from build123d import *

# Parameters (mm, degrees)
BOSS_EXTRUDE1_DEPTH = 15
HOLE1_D             = 51
HOLE2_D             = 14
HOLE2_DEPTH         = 15
HOLE3_D             = 20
HOLE3_DEPTH         = 15
FILLET1_R           = 2
CHAMFER1_SIZE       = 0.81
CHAMFER2_SIZE       = 2


with BuildPart() as part:
    # Sketch1 → Boss-Extrude1 (new body)
    with BuildSketch(Plane(origin=(0, 0, 0), x_dir=(0, 0, -1), z_dir=(1, 0, 0))):
        with BuildLine():
            Line((-62.994461331, 43.470654948), (-63.982276259, 1.506095834))
            ThreePointArc((-63.982276259, 1.506095834), (-64, 0), (-63.982276259, -1.506095834))
            Line((-63.982276259, -1.506095834), (-62.994461331, -43.470654948))
            ThreePointArc((-62.994461331, -43.470654948), (-57.142135624, -57.142135624), (-43.470654948, -62.994461331))
            Line((-43.470654948, -62.994461331), (-1.506095834, -63.982276259))
            ThreePointArc((-1.506095834, -63.982276259), (0, -64), (1.506095834, -63.982276259))
            Line((1.506095834, -63.982276259), (43.470654948, -62.994461331))
            ThreePointArc((43.470654948, -62.994461331), (57.142135624, -57.142135624), (62.994461331, -43.470654948))
            Line((62.994461331, -43.470654948), (63.982276259, -1.506095834))
            ThreePointArc((63.982276259, -1.506095834), (64, 0), (63.982276259, 1.506095834))
            Line((63.982276259, 1.506095834), (62.994461331, 43.470654948))
            ThreePointArc((62.994461331, 43.470654948), (57.142135624, 57.142135624), (43.470654948, 62.994461331))
            Line((43.470654948, 62.994461331), (1.506095834, 63.982276259))
            ThreePointArc((1.506095834, 63.982276259), (0, 64), (-1.506095834, 63.982276259))
            Line((-1.506095834, 63.982276259), (-43.470654948, 62.994461331))
            ThreePointArc((-43.470654948, 62.994461331), (-57.142135624, 57.142135624), (-62.994461331, 43.470654948))
        make_face()
    extrude(amount=-BOSS_EXTRUDE1_DEPTH)

    # Sketch2 → Revolve1 (revolve)
    with BuildSketch(Plane.XY, mode=Mode.PRIVATE) as revolve1_sk:
        Polygon((-15, 47.5), (-17, 45.5), (-17, 34.5), (-34, 34.5), (-50, 38.787187079), (-50, 76), (-65, 76), (-65, 48), (-67, 46), (-67, 0), (-15, 0), align=None)
    revolve(revolve1_sk.sketch.rotate(Axis((-67, 0, 0), (1, 0, 0)), 180), axis=Axis((-67, 0, 0), (1, 0, 0)))

    # Hole1 (through all)
    with Locations(Plane.ZY.offset(67)):
        with Locations((0, 0)):
            Hole(HOLE1_D / 2)

    # Hole2
    with Locations(Plane(origin=(0, 0, 0), x_dir=(0, 0, -1), z_dir=(1, 0, 0))):
        with Locations((43, 43), (43, -43), (-43, -43), (-43, 43)):
            Hole(HOLE2_D / 2, depth=HOLE2_DEPTH)

    # Hole3
    with Locations(Plane.ZY.offset(65)):
        with Locations((43, 43), (-43, 43), (-43, -43), (43, -43)):
            Hole(HOLE3_D / 2, depth=HOLE3_DEPTH)

    # Fillet1
    fillet1_edges = [part.edges().sort_by_distance(p)[0] for p in [
        (-17, 34.5, 0),
        (-50, 38.787187079, 0),
    ]]
    fillet(fillet1_edges, radius=FILLET1_R)

    # Chamfer1
    chamfer1_edges = [part.edges().sort_by_distance(p)[0] for p in [
        (-15, 0, -64),
        (0, -63.488368795, -22.488375391),
        (0, -64, 0),
        (0, -63.488368795, 22.488375391),
        (-15, 22.488375391, -63.488368795),
        (0, -57.142135624, 57.142135624),
        (0, -22.488375391, 63.488368795),
        (0, 0, 64),
        (0, 22.488375391, 63.488368795),
        (0, 57.142135624, 57.142135624),
        (0, 63.488368795, 22.488375391),
        (0, 64, 0),
        (0, 63.488368795, -22.488375391),
        (0, 57.142135624, -57.142135624),
        (0, 22.488375391, -63.488368795),
        (-15, 57.142135624, -57.142135624),
        (0, 0, -64),
        (0, -22.488375391, -63.488368795),
        (0, -57.142135624, -57.142135624),
        (-15, 63.488368795, -22.488375391),
        (-15, 64, 0),
        (-15, 63.488368795, 22.488375391),
        (-15, 57.142135624, 57.142135624),
        (-15, 22.488375391, 63.488368795),
        (-15, 0, 64),
        (-50, 76, 0),
        (-65, 76, 0),
        (-15, -22.488375391, 63.488368795),
        (-15, -57.142135624, -57.142135624),
        (-15, -57.142135624, 57.142135624),
        (-15, -63.488368795, 22.488375391),
        (-15, -64, 0),
        (-15, -63.488368795, -22.488375391),
        (-15, -22.488375391, -63.488368795),
    ]]
    chamfer(chamfer1_edges, length=CHAMFER1_SIZE)

    # Chamfer2
    chamfer2_edges = [part.edges().sort_by_distance(p)[0] for p in [
        (-67, 0, 25.5),
        (0, 0, 25.5),
    ]]
    chamfer(chamfer2_edges, length=CHAMFER2_SIZE)


solid = part.part
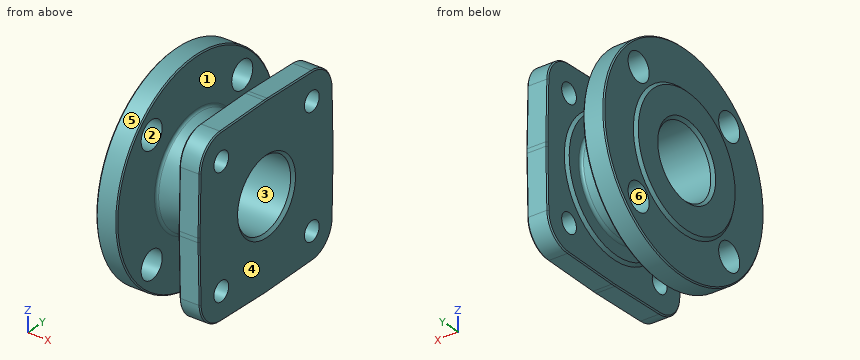
Geometry: final body of the model. Coordinates: model frame, mm. Face numbers are marked on the shaded views. A direction names the side the tool comes from. Coordinates: 2 decimals unless noted, no trailing zeros. Order: outer loops, then holes, each group sorted by start corner. A loop starts at its lowest first (then second) coordinate and runs counter-clockwise, first axis right, second up.
1) Section A-A (x = -4). Return loops of the section in (y, z), then the cut area to 4 significant figures.
Result sheet:
outline: (-63.98, -1.51) - (-62.99, -43.47) arc R20 ccw to (-43.47, -62.99) - (-1.51, -63.98) arc R64 ccw to (1.51, -63.98) - (43.47, -62.99) arc R20 ccw to (62.99, -43.47) - (63.98, -1.51) arc R64 ccw to (63.98, 1.51) - (62.99, 43.47) arc R20 ccw to (43.47, 62.99) - (1.51, 63.98) arc R64 ccw to (-1.51, 63.98) - (-43.47, 62.99) arc R20 ccw to (-62.99, 43.47) - (-63.98, 1.51) arc R64 ccw to start; hole circle Ø14 at (-43, -43); hole circle Ø14 at (-43, 43); hole circle Ø51 at (0, 0); hole circle Ø14 at (43, -43); hole circle Ø14 at (43, 43)
area: 13,050 mm2
2) Draft query along Z for the marked faces 4, 5 and 6. Return one class per face: released by +Z, released by -Z, zero draft, split by the parting line, or undercut.
Result sheet:
face 4: zero draft
face 5: split by the parting line
face 6: undercut
3) Section C-C (x = -60). Return loops of the section in (y, z), then the cut area to 3 significant figures.
Result sheet:
outline: circle Ø152 at (0, 0); hole circle Ø20 at (-43, -43); hole circle Ø20 at (-43, 43); hole circle Ø51 at (0, 0); hole circle Ø20 at (43, -43); hole circle Ø20 at (43, 43)
area: 14,800 mm2
4) Set-up query: the marked faces 1, 2 and 3. Return all of +Z, -Z, +X, -X, +Y, -Y with unobstructed straight access to the full face (end or side cutting, diameter ignored); none if empty.
Result sheet:
face 1: none
face 2: -X
face 3: +X, -X
5) Ray query, probe 1 along Y at (x, z) = (-6.5, 43); probe 2 along X at (y, z) = (-0.5, 63); probe 3 along Y at (x, z) = (-58, 43). Return the intervals inside material, ascending.
Result sheet:
probe 1: y = -63.01 to -50, -36 to 36, 50 to 63.01
probe 2: x = -65 to -50, -15 to 0
probe 3: y = -62.67 to -53, -33 to 33, 53 to 62.67
6) Section B-B (x = -25). Return loops of the section in (y, z).
Result sheet:
outline: circle Ø69 at (0, 0); hole circle Ø51 at (0, 0)
7) First-contact query: P1, Ø10, axis at x = -56, y = 42.5, coming from the +Z side; P2, Ø18, axis at y = -43, z = -43, coming from the -X side; P3, Ø10, axis at y = -21.5, z = 36, coming from the +X side; P4, Ø12, axis at y = 43, z = -43, coming from the -X side. Flat tips, straight axial feed; report the tip coordinate or a pass-through.
Result sheet:
P1: stops at z = 66.1
P2: stops at x = -15
P3: stops at x = 0
P4: passes through
